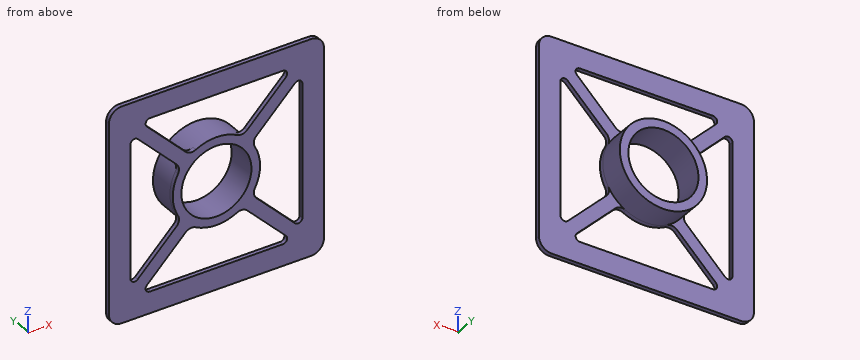
from build123d import *

# Parameters (mm, degrees)
SKETCH1_W           = 50
SKETCH1_H           = 50
SKETCH1_R           = 8.15
BASE_FLANGE1_DEPTH  = 1
FILLET1_R           = 3
FILLET2_R           = 1
FILLET3_R           = 2
BOSS_EXTRUDE1_START = 6
SKETCH2_R           = 10.15
SKETCH2_R_2         = 8.15
BOSS_EXTRUDE1_DEPTH = 6


# Sheet-metal steps are written as plain solids
with BuildPart() as part:
    # Sketch1 → Base-Flange1 (new body)
    with BuildSketch(Plane(origin=(0, 0, 0), x_dir=(1, 0, 0), z_dir=(0, 1, 0))):
        Rectangle(SKETCH1_W, SKETCH1_H)
        with Locations(Location((0, 0, 0), (0, 0, 270))):
            Circle(SKETCH1_R, mode=Mode.SUBTRACT)
        with BuildLine():
            Line((20, 17.878679656), (20, -17.878679656))
            Line((20, -17.878679656), (8.15898744, -6.037667096))
            ThreePointArc((8.15898744, -6.037667096), (10.15, 0), (8.15898744, 6.037667096))
            Line((8.15898744, 6.037667096), (20, 17.878679656))
        make_face(mode=Mode.SUBTRACT)
        with BuildLine():
            Line((17.878679656, -20), (-17.878679656, -20))
            Line((-17.878679656, -20), (-6.037667096, -8.15898744))
            ThreePointArc((-6.037667096, -8.15898744), (0, -10.15), (6.037667096, -8.15898744))
            Line((6.037667096, -8.15898744), (17.878679656, -20))
        make_face(mode=Mode.SUBTRACT)
        with BuildLine():
            Line((-20, -17.878679656), (-20, 17.878679656))
            Line((-20, 17.878679656), (-8.15898744, 6.037667096))
            ThreePointArc((-8.15898744, 6.037667096), (-10.15, 0), (-8.15898744, -6.037667096))
            Line((-8.15898744, -6.037667096), (-20, -17.878679656))
        make_face(mode=Mode.SUBTRACT)
        with BuildLine():
            Line((-17.878679656, 20), (17.878679656, 20))
            Line((17.878679656, 20), (6.037667096, 8.15898744))
            ThreePointArc((6.037667096, 8.15898744), (0, 10.15), (-6.037667096, 8.15898744))
            Line((-6.037667096, 8.15898744), (-17.878679656, 20))
        make_face(mode=Mode.SUBTRACT)
    extrude(amount=-BASE_FLANGE1_DEPTH)

    # Fillet1
    fillet1_edges = [part.edges().sort_by_distance(p)[0] for p in [
        (25, -0.5, 25),
        (-25, -0.5, 25),
        (-25, -0.5, -25),
        (25, -0.5, -25),
    ]]
    fillet(fillet1_edges, radius=FILLET1_R)

    # Fillet2
    fillet2_edges = [part.edges().sort_by_distance(p)[0] for p in [
        (17.878679656, -0.5, 20),
        (-17.878679656, -0.5, 20),
        (20, -0.5, -17.878679656),
        (20, -0.5, 17.878679656),
        (17.878679656, -0.5, -20),
        (-17.878679656, -0.5, -20),
        (-20, -0.5, -17.878679656),
        (-20, -0.5, 17.878679656),
    ]]
    fillet(fillet2_edges, radius=FILLET2_R)

    # Fillet3
    fillet3_edges = [part.edges().sort_by_distance(p)[0] for p in [
        (-6.037667096, -0.5, 8.15898744),
        (6.037667096, -0.5, 8.15898744),
        (8.15898744, -0.5, -6.037667096),
        (8.15898744, -0.5, 6.037667096),
        (6.037667096, -0.5, -8.15898744),
        (-6.037667096, -0.5, -8.15898744),
        (-8.15898744, -0.5, -6.037667096),
        (-8.15898744, -0.5, 6.037667096),
    ]]
    fillet(fillet3_edges, radius=FILLET3_R)

    # Sketch2 → Boss-Extrude1 (add)
    with BuildSketch(Plane(origin=(0, 0, 0), x_dir=(1, 0, 0), z_dir=(0, 1, 0)).offset(BOSS_EXTRUDE1_START)):
        with Locations(Location((0, 0, 0), (0, 0, 270))):
            Circle(SKETCH2_R)
        with Locations(Location((0, 0, 0), (0, 0, 270))):
            Circle(SKETCH2_R_2, mode=Mode.SUBTRACT)
    extrude(amount=-BOSS_EXTRUDE1_DEPTH)


solid = part.part
Here's how the part is built. I have some questions about the finished solid (model axes, mm). Coordinates: 2 decimals unless noted, no trailing zeros. Write each loop counter-clockwise with the first axis right and the second up, starting at its lowest first coordinate (ties: lowest second). Pieces come first, ordered by that corner, then holes.
Item 1: Will these pins go through, and if not, where does the flat tip stop? pin 1 (12 mm diameter, centred on x = 7.5, z = 7.5, fed in from +Y); pin 2 (1.5 mm diameter, centred on x = 16.5, z = -13, fed in from -Y); pin 3 (5 mm diameter, centred on x = 17, z = 19, fed in from +Y).
Item 2: If I drill on line 1 (Y direction, x = -8.5, z = -22.5); line 2 (Z direction, x = -7, y = 0.5); line 3 (X direction, y = 2.25, z = 0), over which ranges is the centre line in solid material (lowest first)?
Item 3: I want a section at A-A on z = 0. Write out the boundary of the cut face in (x, y).
Item 4: I want a section at B-B on z = -19. Write out the boundary of the cut face in (x, y), and give its area (3 significant figures).
Item 5: I want a section at C-C on y = 1.25. Write out the boundary of the cut face in (x, z).
Item 6: I want a section at D-D on z = 6. Write out the boundary of the cut face in (x, y).
Findings below:
1. pin 1: stops at y = 6
1. pin 2: passes through
1. pin 3: stops at y = 0
2. line 1: y = -1 to 0
2. line 2: z = -7.35 to -4.17, 4.17 to 7.35
2. line 3: x = -10.15 to -8.15, 8.15 to 10.15
3. outline: (-25, -1) - (-20, -1) - (-20, 0) - (-25, 0) - close; (-10.15, -1) - (-8.15, -1) - (-8.15, 6) - (-10.15, 6) - close; (8.15, -1) - (10.15, -1) - (10.15, 6) - (8.15, 6) - close; (20, -1) - (25, -1) - (25, 0) - (20, 0) - close
4. outline: (-25, -1) - (-16.46, -1) - (-16.46, 0) - (-25, 0) - close; (16.46, -1) - (25, -1) - (25, 0) - (16.46, 0) - close
4. area: 17.1 mm2
5. outline: circle Ø20.3 at (0, 0); hole circle Ø16.3 at (0, 0)
6. outline: (-25, -1) - (-20, -1) - (-20, 0) - (-25, 0) - close; (-8.72, -1) - (-5.52, -1) - (-5.52, 6) - (-8.19, 6) - (-8.19, 0) - (-8.72, 0) - close; (5.52, -1) - (8.72, -1) - (8.72, 0) - (8.19, 0) - (8.19, 6) - (5.52, 6) - close; (20, -1) - (25, -1) - (25, 0) - (20, 0) - close
